Read the model definition and answer for the solid it produces. Units are mm, in the model's axes. Face numbers are marked on the shaded views. Coordinates: 2 decimals unless noted, no trailing zeros. Write each loop counter-clockwise with the first axis right and the second up, starting at its lowest first coordinate (ties: lowest second). Pieces come first, ordered by that corner, then holes.
(1) The part is cut by section D-D, the plane y = -4.5. Determine the outline of the cut face in (x, z).
(2) Straight lines are drawn through the part: line 1 along X through (y, z) = (135.5, 0); line 2 along Z through (x, y) = (-18, 148.5). For each, find the intervals that lie inside material, in ascending order.
(3) Given pin 1 (2 mm diameter, centred on x = -3.5, y = 127, fed in from +Z); pin 2 (1 mm diameter, centred on x = -18.5, y = 126, fed in from -Z); pin 3 (3 mm diameter, centred on x = -13, z = 12.5, fed in from -Y), each flat-ended and moving along its own axis, determine where each tip first touches the part or whether it passes through.
(4) The part is cut by section B-B, the plane y = 161. Determine the outline of the cut face in (x, z).
(5) Determine the mould class of the marked faces 1 and 2 for opening direction Z: pulls with the +Z half, pulls with the -Z half, needs draft (parallel to the pull), parting line crosses it, or undercut.
(6) The part is cut by section A-A, the plane x = 0. Determine the outline of the cut face in (y, z).
(7) The part is cut by section C-C, the plane z = 0. Determine the outline of the cut face in (x, y).
Autodesk Fusion 360 part; units mm, degrees
sphere "SpherePrimitive1" add diameter 80 placed x (1, 0, 0) y (0, 0, -1) z (0, 1, 0) at (0, 0, 0)
sketch "Sketch2" plane through (0, 0, 0) normal (0, 1, 0) x (1, 0, 0)
  circle A0 centre (0, 0) radius 25
  dimension "d2" = 50
extrude "Extrude1" add sketch "Sketch2" along normal blind 200
hole "Hole1" at (0, 200, 0) direction (0, -1, 0) diameter 42 depth 170 tip angle 180
extrude "Extrude2" cut 1 faces at (23.554, 200, 1.7651) along direction (0, -1, 0) blind 20
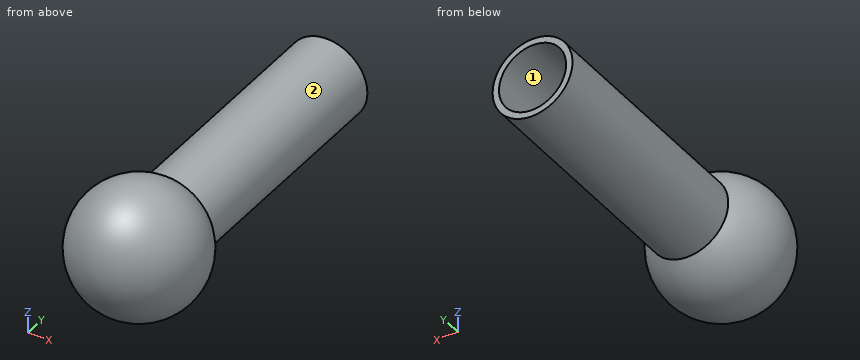
Computed:
1. outline: circle Ø79.49 at (0, 0)
2. line 1: x = -25 to -21, 21 to 25
2. line 2: z = -17.35 to -10.82, 10.82 to 17.35
3. pin 1: stops at z = 24.87
3. pin 2: stops at z = -17.35
3. pin 3: stops at y = -36.42
4. outline: circle Ø50 at (0, 0); hole circle Ø42 at (0, 0)
5. face 1: undercut
5. face 2: parting line crosses it
6. outline: (30, -21) - (30, 21) - (180, 21) - (180, 25) - (31.22, 25) arc R40 ccw (long way) to (31.22, -25) - (180, -25) - (180, -21) - close
7. outline: (-25, 31.22) arc R40 ccw (long way) to (25, 31.22) - (25, 180) - (21, 180) - (21, 30) - (-21, 30) - (-21, 180) - (-25, 180) - close
